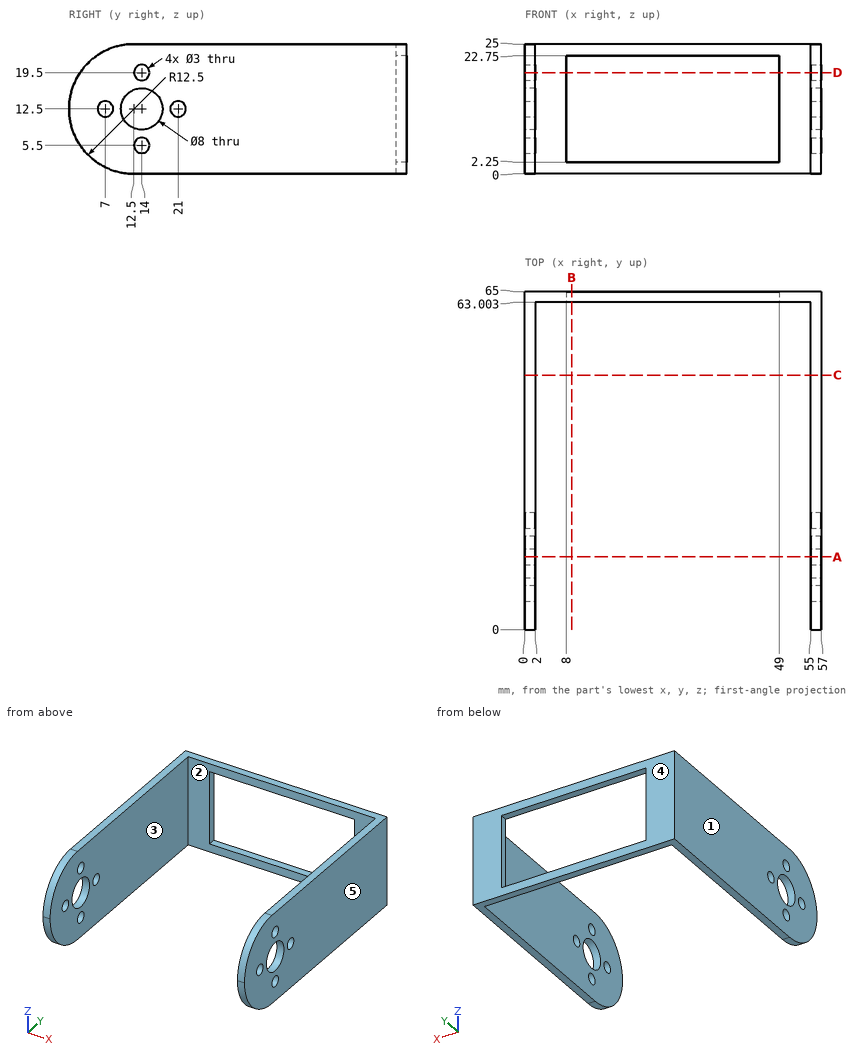
Study the drawing (mm; zero at the part's minimum x, y, z) and answer. A direction names the side the tool comes from. Give positions to 0.01 mm unless a question says otherwise; leave off trailing zeros. Write each loop counter-clockwise with the first axis right and the second up, starting at its lowest first coordinate (ties: lowest second). Pieces come first, ordered by that corner, then holes.
(1) Which of the six approach directions +Z, -Z, +X, -X, +Y, -Y give full straight-line access (tool end or side, diameter ignored) to the marked faces 1 and 2?
Final values:
face 1: +Z, -Z, -X, +Y, -Y
face 2: +Z, -Z, -Y
(2) Flat-ended cylindrical pins translate along their axes: pin 1 Ø10 at (x, z) = (37.5, 10.5) entering from -Y; pin 2 Ø4 at (y, z) = (14, 5.5) entering from +X; pin 3 Ø3 at (x, z) = (7.5, 20.5) entering from -Y. Find the tip coordinate at first contact, or state that the pin passes through.
Final values:
pin 1: passes through
pin 2: stops at x = 57
pin 3: stops at y = 63
(3) A straight line is drawn through the part: line 1 (X direction, y = 5.5, z = 18). Find the intervals that lie inside material, in ascending order.
Final values:
line 1: x = 0 to 2, 55 to 57
(4) The part is cut by section B-B on x = 9. Write down the section's boundary in (y, z).
Final values:
outline: (63, 0) - (65, 0) - (65, 2.25) - (63, 2.25) - close; (63, 22.75) - (65, 22.75) - (65, 25) - (63, 25) - close
(5) The part is cut by section D-D on z = 19.5. Write down the section's boundary in (x, y).
Final values:
outline: (0, 2.14) - (2, 2.14) - (2, 12.5) - (0, 12.5) - close; (0, 15.5) - (2, 15.5) - (2, 63) - (8, 63) - (8, 65) - (0, 65) - close; (49, 63) - (55, 63) - (55, 15.5) - (57, 15.5) - (57, 65) - (49, 65) - close; (55, 2.14) - (57, 2.14) - (57, 12.5) - (55, 12.5) - close
(6) The part is cut by section C-C on y = 49. Write down the section's boundary in (x, z).
Final values:
outline: (0, 0) - (2, 0) - (2, 25) - (0, 25) - close; (55, 0) - (57, 0) - (57, 25) - (55, 25) - close
(7) The mould has two halves that part along X. Classify the marked faces 3, 4 and 5: pulls with the +X half, pulls with the -X half, needs draft (parallel to the pull), parting line crosses it, or undercut.
Final values:
face 3: undercut
face 4: needs draft
face 5: pulls with the +X half
(8) The part is cut by section A-A on y = 14. Count the separate pieces of the cut face and the enclosed holes in it.
Final values:
separate pieces: 8
enclosed holes: 0
